Input: part model. Units: mm. Frame: model coordinates. Give positions to 0.01 mm unless a question says otherwise; leave off trailing zeros. Order: outer loops, then holes, each group sorted by start corner. A loop starts at its lowest first (then second) coordinate and runs counter-clockwise, first axis right, second up. Notation, with made-up numbers: M 60.5,-16 L 107.5,-16 A25 ccw 107.5,22 Z; hole C 25,1.5 d2. An arc over 180 degrees is marked long. Use a Markdown table: item, result.
from build123d import *

# Parameters (mm, degrees)
BOX011_W      = 634
BOX011_H      = 20
BOX011_DEPTH  = 15
BOX010_W      = 634
BOX010_H      = 20
BOX010_DEPTH  = 15
SKETCH009_R   = 2.05
HOLE004_DEPTH = 1270.486422
SKETCH018_R   = 2.05
HOLE011_DEPTH = 1288.986422


with BuildPart() as reference_cube_cut:
    # Box011 → Box011 (new body)
    with BuildSketch(Plane(origin=(1.5, 1.5, 1.5), x_dir=(1, 0, 0), z_dir=(0, 0, 1))):
        with Locations((317, 10)):
            Rectangle(BOX011_W, BOX011_H)
    extrude(amount=BOX011_DEPTH)


with BuildPart() as bottom_body:
    # Box010 → Box010 (new body)
    with BuildSketch(Plane(origin=(1.5, 0, 0), x_dir=(1, 0, 0), z_dir=(0, 0, 1))):
        with Locations((317, 10)):
            Rectangle(BOX010_W, BOX010_H)
    extrude(amount=BOX010_DEPTH)

    # Cut005: cut reference_cube_cut
    add(reference_cube_cut.part, mode=Mode.SUBTRACT)


with BuildPart() as bottom_body_1:
    # Cut005 placement: moved
    add(bottom_body.part.moved(Location((1.5, 1.5, 23))))


with BuildPart() as bottom_body_2:
    # BaseFeature003 placement: moved
    add(bottom_body_1.part.moved(Location((-1.5, -1.5, -23))))

    # Sketch009 → Hole004 (cut, through all)
    with BuildSketch(Plane.XY.offset(1.5)):
        with Locations((10.75, 10.75)):
            Circle(SKETCH009_R)
    hole004 = extrude(amount=-HOLE004_DEPTH, mode=Mode.SUBTRACT)

    # Mirrored002: Hole004 across Sketch009 Axis0
    add(hole004.mirror(Plane(origin=(318.5, 20, 1.5), x_dir=(0, 0, 1), z_dir=(1, 0, 0))), mode=Mode.SUBTRACT)

    # Sketch018 → Hole011 (cut, through all)
    with BuildSketch(Plane.XZ):
        with Locations((10, 8.25)):
            Circle(SKETCH018_R)
    hole011 = extrude(amount=-HOLE011_DEPTH, mode=Mode.SUBTRACT)

    # Mirrored006: Hole011 across Sketch018 Axis0
    add(hole011.mirror(Plane(origin=(318.5, 0, 15), x_dir=(0, -1, 0), z_dir=(1, 0, 0))), mode=Mode.SUBTRACT)


with BuildPart() as bottom_body_3:
    # Body003 placement: moved
    add(bottom_body_2.part.moved(Location((1.5, 1.5, 21.5))))


with BuildPart() as front_bottom_mirror:
    # Part__Mirroring004: instance of bottom_body
    add(bottom_body_3.part.mirror(Plane(origin=(490, 4e-06, 29), x_dir=(1, 0, 0), z_dir=(0, 1, 0))))


with BuildPart() as front_bottom_mirror_1:
    # Part__Mirroring004 placement: moved
    add(front_bottom_mirror.part.moved(Location((0, 320, 0))))


solid = front_bottom_mirror_1.part
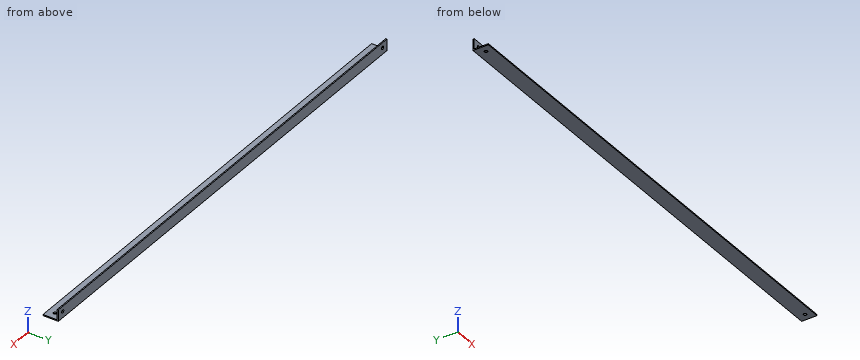
1) First-contact query: pin 1 Ø5 at (x, z) = (565, 29.5) entering from -Y; pin 2 Ø3.5 at (x, y) = (12.25, 307.75) entering from -Z. Flat tips, straight axial feed; report the tip coordinate or a pass-through.
Response values:
| item | result |
|---|---|
| pin 1 | stops at y = 317 |
| pin 2 | passes through |
2) Cut plane B-B on y = 302.5. Return loops of the section in (x, z).
Response values:
| item | result |
|---|---|
| outline | M 3,21.5 L 637,21.5 L 637,23 L 3,23 Z |
3) Material intervals for line 1 (Y direction, x = 627.75, z = 22.45); line 2 (Z direction, x = 11.5, y = 317.95); line 3 (Y direction, x = 450, z = 28), sorted ascending. Write a range as from..to.
Response values:
| item | result |
|---|---|
| line 1 | y = 298.5..305.7, 309.8..318.5 |
| line 2 | z = 21.5..27.7, 31.8..36.5 |
| line 3 | y = 317..318.5 |
4) Cut plane A-A on x = 195. Return loops of the section in (y, z), and give its area (4 significant figures).
Response values:
| item | result |
|---|---|
| outline | M 298.5,21.5 L 318.5,21.5 L 318.5,36.5 L 317,36.5 L 317,23 L 298.5,23 Z |
| area | 50.25 mm² |
